Read the model definition and answer for the solid it produces. Units are mm, in the model's axes. Face numbers are marked on the shaded views. A direction names the side the tool comes from. Coordinates: 2 decimals unless noted, no trailing zeros. Write each loop counter-clockwise with the first axis right and the second up, starting at its lowest first coordinate (ties: lowest second). Pieces come first, ordered by that corner, then holes.
Item 1: Straight lines are drawn through the part: probe 1 along X at (y, z) = (1.9, 0); probe 2 along Z at (x, y) = (0.5, 5); probe 3 along Y at (x, z) = (-3, -5). For each, find the intervals that lie inside material, in ascending order.
Item 2: A tool of negligible diameter and unlimited length cuts with its end or side. For the marked faces 3, 4 and 5, from which of +Z, -Z, +X, -X, +Y, -Y can it reach the whole face along a straight path? Write none if from no direction.
Item 3: Section C-C (z = 3.81) is taken. Give the vertices of the cut face in (x, y), then the cut area to 3 significant figures.
Item 4: Section D-D (x = 1.75) is taken. Give the vertices of the cut face in (y, z) (1 decimal), then the cut area to 3 significant figures.
Item 5: Section A-A (z = 0) is taken. State how many separate pieces and enclosed holes the cut face has, then the cut area to 3 significant figures.
Item 6: Section B-B (x = -0.25) is taken. Give the vertices of the cut face in (y, z) (1 decimal).
Item 7: Determine the mould class of the marked faces 1 and 2 for opening direction Y: released by +Y, released by -Y, zero draft, split by the parting line, or undercut.
Item 8: Each of these flat-tipped pins is pushed along its axis until it touches: P1, Ø2, axis at x = 0, y = 5, coming from the -Z side; P2, Ø1.3, axis at y = 6, z = 0.5, coming from the -X side; P3, Ø0.8, axis at y = 6, z = 0, coming from the +X side. Where does it stop, or does it pass through?
from build123d import *

# Parameters (mm, degrees)
SKETCH1_R               = 6.35
BUTTON_DEPTH            = 2.54
ONE_LEG_DEPTH           = 6.35
MOAR_LEGS_COUNT         = 4
SKETCH3_R               = 6.35
BUTTON_BOTTOM_DEPTH     = 2.54
BUTTON_TOP_FACE_RADIUS  = 6.35
BUTTON_TOP_HEIGHT       = 2.54
SKETCH5_R               = 0.635
SKETCH6_R               = 1.27
RECESS_FOR_SPRING_DEPTH = 0.762


with BuildPart() as part:
    # Sketch1 → button (new body)
    with BuildSketch(Plane(origin=(0, 0, 0), x_dir=(1, 0, 0), z_dir=(0, 1, 0))):
        with Locations(Location((0, 0, 0), (0, 0, 270))):
            Circle(SKETCH1_R)
    extrude(amount=BUTTON_DEPTH)

    # Sketch2 → one leg (add)
    with BuildSketch(Plane(origin=(0, 2.54, 0), x_dir=(1, 0, 0), z_dir=(0, 1, 0))):
        with BuildLine():
            Line((-1.27, -3.048), (1.27, -3.048))
            ThreePointArc((1.27, -3.048), (2.032, -3.81), (1.27, -4.572))
            Line((1.27, -4.572), (-1.27, -4.572))
            ThreePointArc((-1.27, -4.572), (-2.032, -3.81), (-1.27, -3.048))
        make_face()
    one_leg = extrude(amount=ONE_LEG_DEPTH)

    # moar legs: one leg ×4 about axis
    moar_legs_axis = Axis((0, 0, 0), (0, 1, 0))
    for i in range(1, MOAR_LEGS_COUNT):
        add(one_leg.rotate(moar_legs_axis, i * 360 / MOAR_LEGS_COUNT))

    # Sketch3 → button bottom (add)
    with BuildSketch(Plane(origin=(0, 8.89, 0), x_dir=(1, 0, 0), z_dir=(0, 1, 0))):
        with Locations(Location((0, 0, 0), (0, 0, 270))):
            Circle(SKETCH3_R)
    extrude(amount=BUTTON_BOTTOM_DEPTH)

    # button top: a dome of height H over a round flat face of radius A is a cap of a sphere of radius (A * A + H * H) / (2 * H)
    button_top_r = (BUTTON_TOP_FACE_RADIUS * BUTTON_TOP_FACE_RADIUS + BUTTON_TOP_HEIGHT * BUTTON_TOP_HEIGHT) / (2 * BUTTON_TOP_HEIGHT)
    button_top_base = Plane((0, 0, 0), z_dir=(0, -1, 0))
    with Locations(button_top_base.offset(BUTTON_TOP_HEIGHT - button_top_r)):
        button_top_ball = Sphere(button_top_r, mode=Mode.PRIVATE)
    add(split(button_top_ball, bisect_by=button_top_base, keep=Keep.TOP, mode=Mode.PRIVATE))

    # handle for linkage: sweep along a path in Sketch4
    with BuildLine(Plane.XY) as handle_for_linkage_path:
        Line((-3.689676867, 11.43), (-3.689676867, 13.163817949))
        ThreePointArc((-3.689676867, 13.163817949), (-3.317702479, 14.061843561), (-2.419676867, 14.433817949))
        Line((-2.419676867, 14.433817949), (2.419676867, 14.433817949))
        ThreePointArc((2.419676867, 14.433817949), (3.317702479, 14.061843561), (3.689676867, 13.163817949))
        Line((3.689676867, 13.163817949), (3.689676867, 11.43))
    # Sketch5 → handle for linkage (sweep)
    with BuildSketch(Plane(origin=(0, 11.43, 0), x_dir=(1, 0, 0), z_dir=(0, 1, 0))):
        with Locations((-3.689676867, 0)):
            Circle(SKETCH5_R)
    sweep(path=handle_for_linkage_path.line)

    # Sketch6 → recess for spring (cut)
    with BuildSketch(Plane(origin=(0, 2.54, 0), x_dir=(1, 0, 0), z_dir=(0, 1, 0))):
        with Locations(Location((0, 0, 0), (0, 0, 270))):
            Circle(SKETCH6_R)
    extrude(amount=-RECESS_FOR_SPRING_DEPTH, mode=Mode.SUBTRACT)


solid = part.part
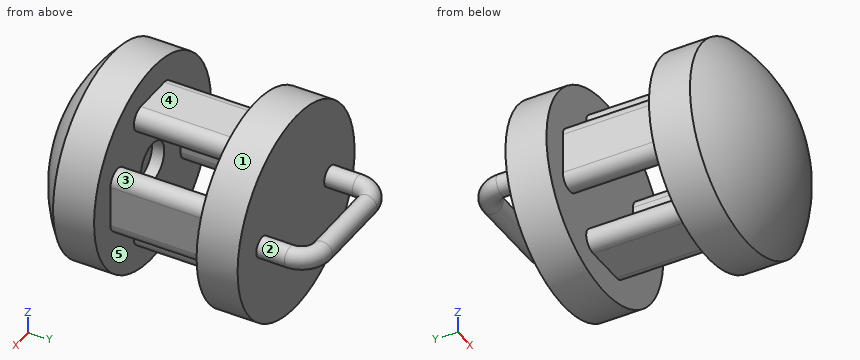
Established:
1. probe 1: x = -6.35 to -1.27, 1.27 to 6.35
1. probe 2: z = -4.57 to -3.05, 3.05 to 4.57
1. probe 3: y = -0.46 to 2.54, 8.89 to 11.43
2. face 3: +Z
2. face 4: +Z, +X, -X
2. face 5: none
3. outline: (-5.08, 0) arc R8.38 ccw to (5.08, 0) - (5.08, 2.54) - (2.03, 2.54) - (2.03, 8.89) - (5.08, 8.89) - (5.08, 11.43) - (-5.08, 11.43) - (-5.08, 8.89) - (-2.03, 8.89) - (-2.03, 2.54) - (-5.08, 2.54) - close
3. area: 89.3 mm2
4. outline: (0, -6.1) - (2.5, -6.1) - (2.5, -4.4) - (8.9, -4.4) - (8.9, -6.1) - (11.4, -6.1) - (11.4, 6.1) - (8.9, 6.1) - (8.9, 4.4) - (2.5, 4.4) - (2.5, 6.1) - (0, 6.1) arc R9 ccw to start; circle Ø1.3 at (14.4, 0); hole (2.5, -3.2) - (8.9, -3.2) - (8.9, 3.2) - (2.5, 3.2) - close
4. area: 98.2 mm2
5. separate pieces: 1
5. enclosed holes: 2
5. area: 120 mm2
6. outline: (0, -6.3) - (2.5, -6.3) - (2.5, -4.6) - (8.9, -4.6) - (8.9, -6.3) - (11.4, -6.3) - (11.4, 6.3) - (8.9, 6.3) - (8.9, 4.6) - (2.5, 4.6) - (2.5, 6.3) - (0, 6.3) arc R9.2 ccw to start; circle Ø1.3 at (14.4, 0); hole (1.8, -1.2) - (2.5, -1.2) - (2.5, -3) - (8.9, -3) - (8.9, 3) - (2.5, 3) - (2.5, 1.2) - (1.8, 1.2) - close
7. face 1: zero draft
7. face 2: undercut
8. P1: stops at z = -4.57
8. P2: stops at x = -4.57
8. P3: stops at x = 4.57
